Work out the finished part from the listing and answer in its coordinate system (mm). A direction names the side the tool comes from. Coordinates: 2 decimals unless noted, no trailing zeros. Order: outer loops, then holes, each group sorted by start corner. A loop starts at its lowest first (then second) coordinate and runs counter-clockwise, first axis right, second up. Notation, with made-up numbers: M 14.5,78 L 43.5,78 A15 ccw 43.5,105 Z; hole C 26.25,73.25 d6. An arc over 180 degrees is marked long. Use a Markdown table: item, result.
from build123d import *

# Parameters (mm, degrees)
F0_W     = 100
F0_H     = 35
F1_DEPTH = 3
F2_W     = 2
F2_H     = 35
F3_DEPTH = 3.001


with BuildPart() as f1:
    # F0 (on Top) → F1 (new body)
    with BuildSketch(Plane.XY):
        Rectangle(F0_W, F0_H)
    extrude(amount=F1_DEPTH)

    # F2 (on face) → F3 (cut, through all)
    with BuildSketch(Plane.XY.offset(3)):
        with Locations((47, -8)):
            Rectangle(F2_W, F2_H)
        with Locations((43, -8)):
            Rectangle(F2_W, F2_H)
        with Locations((39, -8)):
            Rectangle(F2_W, F2_H)
        with Locations((35, -8)):
            Rectangle(F2_W, F2_H)
        with Locations((31, -8)):
            Rectangle(F2_W, F2_H)
        with Locations((27, -8)):
            Rectangle(F2_W, F2_H)
        with Locations((23, -8)):
            Rectangle(F2_W, F2_H)
        with Locations((19, -8)):
            Rectangle(F2_W, F2_H)
        with Locations((15, -8)):
            Rectangle(F2_W, F2_H)
        with Locations((11, -8)):
            Rectangle(F2_W, F2_H)
        with Locations((7, -8)):
            Rectangle(F2_W, F2_H)
        with Locations((3, -8)):
            Rectangle(F2_W, F2_H)
        with Locations((-1, -8)):
            Rectangle(F2_W, F2_H)
        with Locations((-5, -8)):
            Rectangle(F2_W, F2_H)
        with Locations((-9, -8)):
            Rectangle(F2_W, F2_H)
        with Locations((-13, -8)):
            Rectangle(F2_W, F2_H)
        with Locations((-17, -8)):
            Rectangle(F2_W, F2_H)
        with Locations((-21, -8)):
            Rectangle(F2_W, F2_H)
        with Locations((-25, -8)):
            Rectangle(F2_W, F2_H)
        with Locations((-29, -8)):
            Rectangle(F2_W, F2_H)
    extrude(amount=-F3_DEPTH, mode=Mode.SUBTRACT)


solid = f1.part
1. Section B-B on x = 39 is taken. Determine the outline of the cut face in (y, z), then the cut area to 3 significant figures.
Answers below:
| item | result |
|---|---|
| outline | M 9.5,0 L 17.5,0 L 17.5,3 L 9.5,3 Z |
| area | 24.0 mm² |
2. Find the intervals of material crossed by probe 1 along Y at (x, z) = (-5, 1.9), in increasing order.
Answers below:
| item | result |
|---|---|
| probe 1 | 9.5 to 17.5 |
3. For faces 4 (the face through (9, -17.5, 1)), 5 (the face through (20, -4, 2)), determine the directions among +Z, -Z, +X, -X, +Y, -Y from which every point of the face is accessible in a straight line to the end or side of a thin tool.
Answers below:
| item | result |
|---|---|
| face 4 | +Z, -Z, +X, -X, -Y |
| face 5 | +Z, -Z, -Y |
4. Section A-A on y = 4.5 is taken. Give the number of separate pieces and of enclosed holes in the cut face, then the cut area to 3 significant figures.
Answers below:
| item | result |
|---|---|
| separate pieces | 21 |
| enclosed holes | 0 |
| area | 180 mm² |
5. For a pull along X with two mould halves and no side action, classify faces 1 (the face through (50, 0, 1)), 2 (the face through (2, -4, 2)), 3 (the face through (33, -17.5, 1)) as +X half, -X half, draft (parallel to the pull), parting line (faces both ways), or undercut.
Answers below:
| item | result |
|---|---|
| face 1 | +X half |
| face 2 | undercut |
| face 3 | draft |
